Answer from the drawing. Dimensions are ordinates in mm from the lowest x, y and z of the part. A direction names the side the tool comes from. Coordinates: 2 decimals unless noted, no trailing zeros. Order: outer loops, then holes, each group sorted by start corner. A loop starts at its lowest first (then second) coordinate and runs counter-clockwise, first axis right, second up. Notation, with made-up numbers: M 10.25,2 L 21.25,2 A17 ccw 21.25,17 Z; hole C -35,-15 d9. An arc over 180 degrees is marked long. Write each question's results on one line, items separated by ' | '.
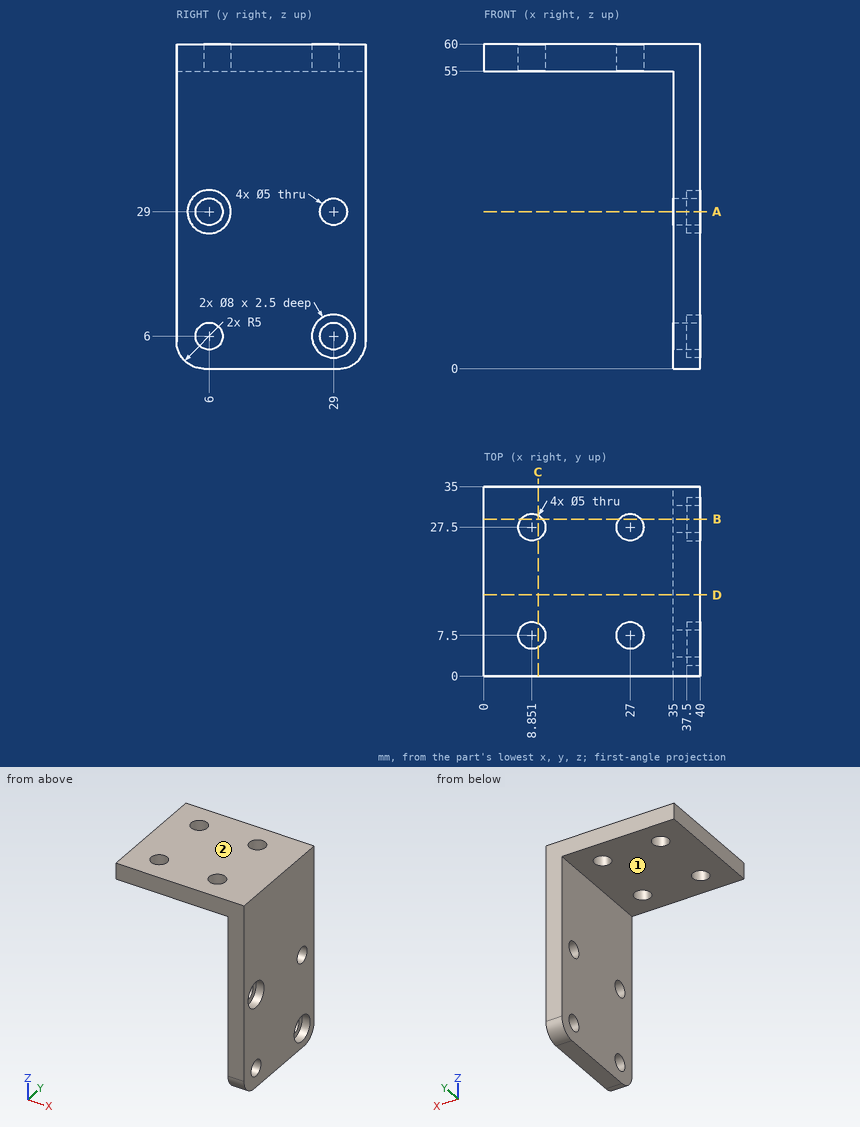
(1) The part is cut by section A-A, the plane z = 29. Write down the section's boundary in (x, y).
Conclusion:
outline: M 35,0 L 40,0 L 40,2 L 37.5,2 L 37.5,3.5 L 35,3.5 Z; M 35,8.5 L 37.5,8.5 L 37.5,10 L 40,10 L 40,26.5 L 35,26.5 Z; M 35,31.5 L 40,31.5 L 40,35 L 35,35 Z
(2) Straight lines are drawn through the part: line 1 (Y direction, x = 37.65, z = 6); line 2 (X direction, y = 7, z = 57); line 3 (Z direction, x = 4, y = 6.5). For each, find the intervals that lie inside material, in ascending order.
Conclusion:
line 1: 0 to 3.5, 8.5 to 25, 33 to 35 | line 2: 0 to 6.4, 11.3 to 24.55, 29.45 to 40 | line 3: 55 to 60
(3) The part is cut by section B-B, the plane y = 29. Write down the section's boundary in (x, z).
Conclusion:
outline: M 0,55 L 6.85,55 L 6.85,60 L 0,60 Z; M 10.85,55 L 25,55 L 25,60 L 10.85,60 Z; M 29,55 L 35,55 L 35,31.5 L 40,31.5 L 40,60 L 29,60 Z; M 35,0 L 40,0 L 40,2 L 37.5,2 L 37.5,3.5 L 35,3.5 Z; M 35,8.5 L 37.5,8.5 L 37.5,10 L 40,10 L 40,26.5 L 35,26.5 Z
(4) The part is cut by section C-C, the plane x = 10. Write down the section's boundary in (y, z), then the cut area to 3 significant figures.
Conclusion:
outline: M 0,55 L 5.28,55 L 5.28,60 L 0,60 Z; M 9.72,55 L 25.28,55 L 25.28,60 L 9.72,60 Z; M 29.72,55 L 35,55 L 35,60 L 29.72,60 Z | area: 131 mm²
(5) Given pin 1 (5 mm diameter, centred on y = 27, z = 48.5, fed in from -X); pin 2 (1.5 mm diameter, centred on x = 32.5, z = 51, fed in from +Y); pin 3 (4 mm diameter, centred on y = 6.5, z = 29.5, fed in from +X); pin 4 (6.5 mm diameter, centred on x = 8.85, y = 7.5, fed in from -Z), each flat-ended and moving along its own axis, determine where each tip first touches the part or whether it passes through.
Conclusion:
pin 1: x = 35 | pin 2: through | pin 3: x = 37.5 | pin 4: z = 55
(6) The part is cut by section D-D, the plane y = 15. Write down the section's boundary in (x, z).
Conclusion:
outline: M 0,55 L 35,55 L 35,0 L 40,0 L 40,60 L 0,60 Z
(7) For the marked faces 1 and 2, determine the directions among +Z, -Z, +X, -X, +Y, -Y from which every point of the face is accessible in a straight line to the end or side of a thin tool.
Conclusion:
face 1: -Z, -X, +Y, -Y | face 2: +Z, +X, -X, +Y, -Y
